Source: three-view drawing plus pictorial views. Frame: mm from the lowest corner of the part. Give positions to 0.01 mm unless a question says otherwise; leave off trailing zeros. Loops run counter-clockwise (first coordinate to the right, second up) from the corner with the lowest first, then second, coordinate; pieces in that order, holes last. Notation, with made-up numbers: (81.5, 34.5) -> (132.5, 34.5) arc R17 ccw to (132.5, 56.5) -> close; hole circle Ø11 at (-10, -19.75). An arc over 180 degrees is marked (long way). One line per item, written item: value. Start each with the question number.
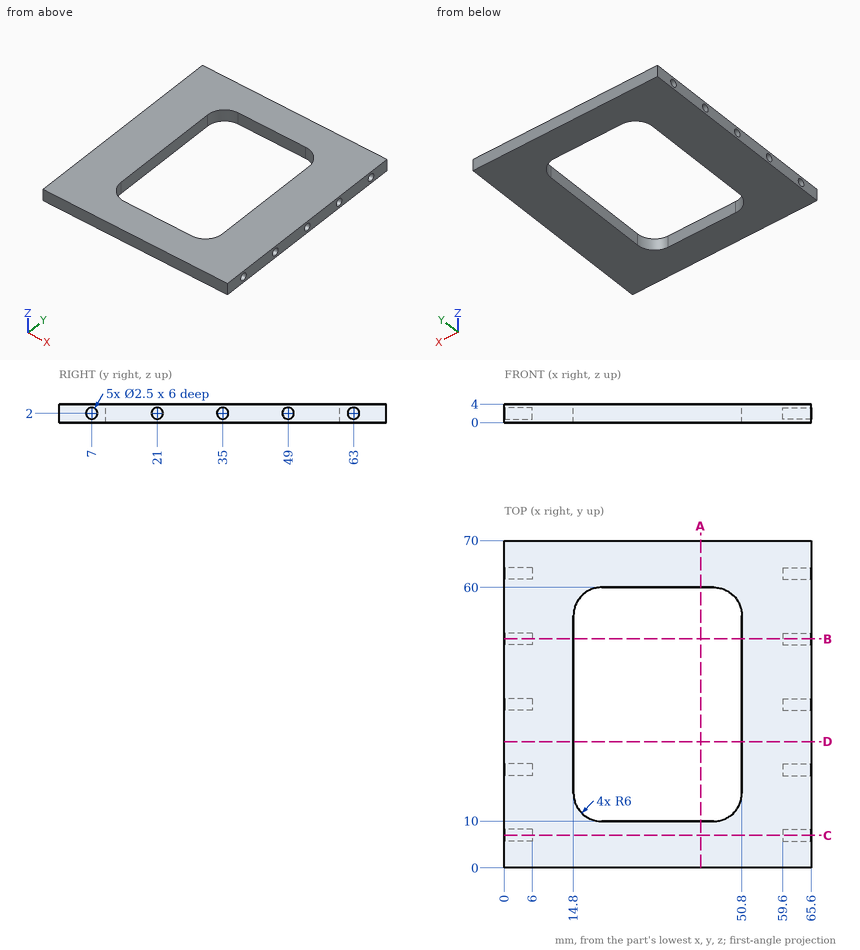
Item 1: Ray query, line 1 along Y through (x, z) = (61.55, 2); line 2 along X through (y, z) = (17, 1.95); line 3 along Y through (x, z) = (35, 0.25). Return the intervals inside material, ascending. Write a range as [from, to].
Item 2: Section D-D, the plane y = 27. Output: boundary loops of the cut face in (x, z), then the cut area to 3 significant figures.
Item 3: Pin query (flat end, axial travel): pin 1 (1.5 mm diameter, centred on y = 7, z = 2, fed in from -X); pin 2 (1 mm diameter, centred on y = 62.5, z = 1.5, fed in from +X). Return the tip coordinate at first contact, or that it passes through.
Item 4: Section A-A, the plane x = 42. Output: boundary loops of the cut face in (y, z), then the cut area to 3 significant figures.
Item 5: Section B-B, the plane y = 49. Output: boundary loops of the cut face in (x, z), then the cut area to 3 significant figures.
Item 6: Section C-C, the plane y = 7. Output: boundary loops of the cut face in (x, z).
Geometry check:
1. line 1: y = [0, 5.75], [8.25, 19.75], [22.25, 33.75], [36.25, 47.75], [50.25, 61.75], [64.25, 70]
1. line 2: x = [0, 14.8], [50.8, 65.6]
1. line 3: y = [0, 10], [60, 70]
2. outline: (0, 0) -> (14.8, 0) -> (14.8, 4) -> (0, 4) -> close; (50.8, 0) -> (65.6, 0) -> (65.6, 4) -> (50.8, 4) -> close
2. area: 118 mm2
3. pin 1: stops at x = 6
3. pin 2: stops at x = 59.6
4. outline: (0, 0) -> (10, 0) -> (10, 4) -> (0, 4) -> close; (60, 0) -> (70, 0) -> (70, 4) -> (60, 4) -> close
4. area: 80.0 mm2
5. outline: (0, 0) -> (14.8, 0) -> (14.8, 4) -> (0, 4) -> (0, 3.25) -> (6, 3.25) -> (6, 0.75) -> (0, 0.75) -> close; (50.8, 0) -> (65.6, 0) -> (65.6, 0.75) -> (59.6, 0.75) -> (59.6, 3.25) -> (65.6, 3.25) -> (65.6, 4) -> (50.8, 4) -> close
5. area: 88.4 mm2
6. outline: (0, 0) -> (65.6, 0) -> (65.6, 0.75) -> (59.6, 0.75) -> (59.6, 3.25) -> (65.6, 3.25) -> (65.6, 4) -> (0, 4) -> (0, 3.25) -> (6, 3.25) -> (6, 0.75) -> (0, 0.75) -> close
